Design review of the part built by this model. Coordinates are the model's own, in mm. A direction names the side the tool comes from. Round coordinates to 2 decimals unless told otherwise and drop trailing zeros. Loops run counter-clockwise (first coordinate to the right, second up) from the corner with the lowest first, then second, coordinate; pieces in that order, holes last. Notation, with made-up numbers: (72.25, 33) -> (124.25, 33) arc R7 ccw to (124.25, 39) -> close; hole circle Ø4 at (34, 57). An arc over 180 degrees is marked (long way). Write each question's results on one line, items separated by ' | '. Start each with the question number.
from build123d import *
from build123d.topology import SkipClean

# Parameters (mm, degrees)
SKETCH_2_R                   = 25
SKETCH_2_R_2                 = 10
EXTRUDE_2_DEPTH              = 2
SKETCH_35_R                  = 13.5
EXTRUDE_3_DEPTH              = 2
SKETCH_36_R                  = 12.5
EXTRUDE_4_DEPTH              = 7
HOLE_WIZARD_M3_1_D           = 3.4
HOLE_WIZARD_M3_1_CBORE_D     = 6.5
HOLE_WIZARD_M3_1_CBORE_DEPTH = 3.4
PATTERN_CIRCULAR_1_COUNT     = 3
PATTERN_CIRCULAR_2_COUNT     = 3
EXTRUDE_START                = 3
SKETCH_53_R                  = 11.5
SKETCH_53_R_2                = 1.25
SKETCH_53_R_3                = 3.25
EXTRUDE_5_DEPTH              = 3
EXTRUDE_START_2              = 7
SKETCH_61_R                  = 10
SKETCH_61_R_2                = 1.7
EXTRUDE_6_DEPTH              = 7
SKETCH_62_R                  = 10
SKETCH_62_R_2                = 9.5
CUT_EXTRUDE_1_DEPTH          = 5
FILLET_1_R                   = 0.1
PATTERN_CIRCULAR_3_COUNT     = 3
SKETCH_82_R                  = 3.25
EXTRUDE_7_DEPTH              = 19
HOLE_WIZARD_M5_1_D           = 5.5
HOLE_WIZARD_M5_1_CBORE_D     = 10
HOLE_WIZARD_M5_1_CBORE_DEPTH = 5.4
PATTERN_CIRCULAR_4_COUNT     = 3


with BuildPart() as part:
    # 스케치2 → 보스-돌출2 (new body)
    with BuildSketch(Plane(origin=(0, 6, 0), x_dir=(1, 0, 0), z_dir=(0, 0, -1))):
        with Locations(Location((0, 6, 0), (0, 0, 180))):
            Circle(SKETCH_2_R)
        with Locations(Location((0, 6, 0), (0, 0, 180))):
            Circle(SKETCH_2_R_2, mode=Mode.SUBTRACT)
    extrude(amount=EXTRUDE_2_DEPTH)

    # 스케치35 → 보스-돌출3 (add)
    with BuildSketch(Plane(origin=(0, 0, -2), x_dir=(-1, 0, 0), z_dir=(0, 0, -1))):
        Circle(SKETCH_35_R)
    extrude(amount=EXTRUDE_3_DEPTH)

    # 스케치36 → 보스-돌출4 (add)
    with BuildSketch(Plane(origin=(0, 0, -4), x_dir=(-1, 0, 0), z_dir=(0, 0, -1))):
        Circle(SKETCH_36_R)
    extrude(amount=EXTRUDE_4_DEPTH)

    # Hole Wizard M3 _ _ _ _ _ _1 (through all)
    with Locations(Plane(origin=(0, 0, -11), x_dir=(-1, 0, 0), z_dir=(0, 0, -1))):
        with Locations((0, 4)):
            hole_wizard_m3_1 = CounterBoreHole(HOLE_WIZARD_M3_1_D / 2, HOLE_WIZARD_M3_1_CBORE_D / 2, HOLE_WIZARD_M3_1_CBORE_DEPTH)

    # 원형 패턴1: Hole Wizard M3 _ _ _ _ _ _1 ×3 about axis
    pattern_circular_1_axis = Axis((0, 0, 0), (0, 0, 1))
    for i in range(1, PATTERN_CIRCULAR_1_COUNT):
        add(hole_wizard_m3_1.rotate(pattern_circular_1_axis, i * 360 / PATTERN_CIRCULAR_1_COUNT), mode=Mode.SUBTRACT)

    # 스케치52 → Hole Wizard M3 _ _ _ _1 2 (revolve, cut)
    with BuildSketch(Plane(origin=(0, -7, -11), x_dir=(0, 1, 0), z_dir=(1, 0, 0))):
        Polygon((0, 0), (0, 5.751075774), (1.25, 5), (1.25, 0), align=None)
    hole_wizard_m3_1_2 = revolve(axis=Axis((0, -7, -17.35), (0, 0, 1)), mode=Mode.SUBTRACT)

    # 원형 패턴2: Hole Wizard M3 _ _ _ _1 2 ×3 about axis
    pattern_circular_2_axis = Axis((0, 0, 0), (0, 0, 1))
    for i in range(1, PATTERN_CIRCULAR_2_COUNT):
        add(hole_wizard_m3_1_2.rotate(pattern_circular_2_axis, i * 360 / PATTERN_CIRCULAR_2_COUNT), mode=Mode.SUBTRACT)

    # 스케치53 → 보스-돌출5 (add)
    with SkipClean():  # the faces are left unmerged after this step: merging them gives an invalid solid
        with BuildSketch(Plane(origin=(0, 0, -11), x_dir=(-1, 0, 0), z_dir=(0, 0, -1)).offset(EXTRUDE_START)):
            Circle(SKETCH_53_R)
            with Locations((6.062177826, 3.5)):
                Circle(SKETCH_53_R_2, mode=Mode.SUBTRACT)
            with Locations((0, -7)):
                Circle(SKETCH_53_R_2, mode=Mode.SUBTRACT)
            with Locations((3.464101615, -2)):
                Circle(SKETCH_53_R_3, mode=Mode.SUBTRACT)
            with Locations((0, 4)):
                Circle(SKETCH_53_R_3, mode=Mode.SUBTRACT)
            with Locations((-3.464101615, -2)):
                Circle(SKETCH_53_R_3, mode=Mode.SUBTRACT)
            with Locations((-6.062177826, 3.5)):
                Circle(SKETCH_53_R_2, mode=Mode.SUBTRACT)
        extrude(amount=-EXTRUDE_5_DEPTH)

    # 스케치61 → 보스-돌출6 (add)
    with BuildSketch(Plane.XY.offset(-2).offset(EXTRUDE_START_2)):
        with Locations(Location((0, 0, 0), (0, 0, 180))):
            Circle(SKETCH_61_R)
        with Locations(Location((-3.464101615, -2, 0), (0, 0, 180))):
            Circle(SKETCH_61_R_2, mode=Mode.SUBTRACT)
        with Locations(Location((3.464101615, -2, 0), (0, 0, 180))):
            Circle(SKETCH_61_R_2, mode=Mode.SUBTRACT)
        with Locations(Location((0, 4, 0), (0, 0, 180))):
            Circle(SKETCH_61_R_2, mode=Mode.SUBTRACT)
    extrude(amount=-EXTRUDE_6_DEPTH)

    # 스케치62 → 컷-돌출1 (cut)
    with BuildSketch(Plane.XY.offset(5)):
        Circle(SKETCH_62_R)
        Circle(SKETCH_62_R_2, mode=Mode.SUBTRACT)
    extrude(amount=-CUT_EXTRUDE_1_DEPTH, mode=Mode.SUBTRACT)

    # 필렛1
    fillet_1_edges = [part.edges().sort_by_distance(p)[0] for p in [
        (-9.5, 0, 0),
        (-9.5, 0, 5),
    ]]
    fillet(fillet_1_edges, radius=FILLET_1_R)

    # 스케치67 → Ø3.0mm 맞춤핀 구멍1 (revolve, cut)
    with BuildSketch(Plane(origin=(0, -7, 5), x_dir=(0, -1, 0), z_dir=(1, 0, 0))):
        Polygon((0, 0), (0, 5.901290929), (1.5, 5), (1.5, 0), align=None)
    f_3_0mm_1 = revolve(axis=Axis((0, -7, 11.35), (0, 0, -1)), mode=Mode.SUBTRACT)

    # 원형 패턴3: Ø3.0mm 맞춤핀 구멍1 ×3 about axis
    pattern_circular_3_axis = Axis((0, 0, 0), (0, 0, 1))
    for i in range(1, PATTERN_CIRCULAR_3_COUNT):
        add(f_3_0mm_1.rotate(pattern_circular_3_axis, i * 360 / PATTERN_CIRCULAR_3_COUNT), mode=Mode.SUBTRACT)

    # 스케치82 → 보스-돌출7 (add)
    with SkipClean():  # the faces are left unmerged after this step: merging them gives an invalid solid
        with BuildSketch(Plane(origin=(0, 0, -14), x_dir=(-1, 0, 0), z_dir=(0, 0, -1))):
            with Locations((0, 4)):
                Circle(SKETCH_82_R)
            with Locations((-3.464101615, -2)):
                Circle(SKETCH_82_R)
            with Locations((3.464101615, -2)):
                Circle(SKETCH_82_R)
        extrude(amount=-EXTRUDE_7_DEPTH)

    # M5 육각 소켓 머리 캡 나사용 카운터보어1 (through all)
    with Locations(Plane(origin=(0, 0, -14), x_dir=(-1, 0, 0), z_dir=(0, 0, -1))):
        with Locations((0, 0)):
            CounterBoreHole(HOLE_WIZARD_M5_1_D / 2, HOLE_WIZARD_M5_1_CBORE_D / 2, HOLE_WIZARD_M5_1_CBORE_DEPTH)

    # 스케치89 → Ø3.0mm 맞춤핀 구멍2 (revolve, cut)
    with BuildSketch(Plane(origin=(0, 8.5, -14), x_dir=(0, 1, 0), z_dir=(1, 0, 0))):
        Polygon((0, 0), (0, 5.901290929), (1.5, 5), (1.5, 0), align=None)
    f_3_0mm_2 = revolve(axis=Axis((0, 8.5, -20.35), (0, 0, 1)), mode=Mode.SUBTRACT)

    # 원형 패턴4: Ø3.0mm 맞춤핀 구멍2 ×3 about axis
    pattern_circular_4_axis = Axis((0, 0, 0), (0, 0, 1))
    for i in range(1, PATTERN_CIRCULAR_4_COUNT):
        add(f_3_0mm_2.rotate(pattern_circular_4_axis, i * 360 / PATTERN_CIRCULAR_4_COUNT), mode=Mode.SUBTRACT)


solid = part.part
1) For faces 1 (the face through (-2.2, -2.2, -8.6)), 2 (the face through (-23.846, 7.509, -0.986)), 3 (the face through (4.575, 3.695, 2.535)), list the 3-axis set-ups (+Z, -Z, +X, -X, +Y, -Y) from which the entire face can be reached by the end or side of a thin tool; tool diameter is ignored.
2) To check wall thickness, follow line 1 (Y direction, x = 0, z = -11.9); line 2 (X direction, y = -4, z = -9.25); line 3 (Y direction, x = 7, z = -10.25). State the ranges of each line that lie inside material, in increasing order. Write a range as from..to.
3) Insertion check: pin 1 (4 mm diameter, centred on x = -6.06, y = 3.5, fed in from +Z); pin 2 (1.5 mm diameter, centred on x = -4.5, z = -0.5, fed in from +Y); pin 3 (5 mm diameter, centred on y = 13.5, z = -7, fed in from +X); pin 4 (2.5 mm diameter, centred on x = 7.36, y = -4.25, fed in from -Z). Each pin has a flat end and moves straight along its axis. Give the tip position at first contact, or say it passes through.
4) Take a section at A-A (z = 2.25). Write out the cut boundary in (x, y).
5) Take a section at B-B (x = -18.5). Write out the cut boundary in (y, z).
6) The part is to be moulded in two halves that separate along Y. For faces 4 (the face through (-0.07, -5.5, 2.54)), 5 (the face through (7.185, -4.442, -8.255)), 6 (the face through (4.38, -8.43, 2.53)), 7 (the face through (-11, -4, -11)), say which applies: +Y half, -Y half, draft (parallel to the pull), parting line (faces both ways), or undercut.
7) Take a section at C-C (z = -6.75). Write out the cut boundary in (x, y) (3 decimals).
8) Take a section at D-D (y = -17). Write out the cut boundary in (x, z).
Geometry check:
1) face 1: -Z | face 2: +Z, -Z | face 3: +Z
2) line 1: y = -11.5..-8.25, -5.75..-5, 5..7, 10..11.5 | line 2: x = -11.84..-8.84, -5.88..-3, 3..5.88, 8.84..11.84 | line 3: y = -10.36..-5.71, -2.79..2.67, 4.33..10.36
3) pin 1: stops at z = 5 | pin 2: stops at y = 24.72 | pin 3: stops at x = 5.94 | pin 4: stops at z = -8.85
4) outline: circle Ø19 at (0, 0); hole circle Ø3 at (-6.06, 3.5); hole circle Ø5.5 at (0, 0); hole circle Ø3 at (0, -7); hole circle Ø3 at (6.06, 3.5)
5) outline: (-16.82, -2) -> (16.82, -2) -> (16.82, 0) -> (-16.82, 0) -> close
6) face 4: undercut | face 5: undercut | face 6: parting line | face 7: draft
7) outline: circle Ø25 at (0, 0); hole circle Ø2.5 at (-6.062, 3.5); hole circle Ø5.5 at (0, 0); hole circle Ø2.5 at (0, -7); hole circle Ø2.5 at (6.062, 3.5)
8) outline: (-18.33, -2) -> (18.33, -2) -> (18.33, 0) -> (-18.33, 0) -> close
